```python
from build123d import *

# Parameters (mm, degrees)
F0_R     = 90
F1_DEPTH = 7.5
F2_R     = 3
F3_DEPTH = 90


with BuildPart() as f1:
    # F0 (on Front) → F1 (new body, symmetric)
    with BuildSketch(Plane.XZ):
        Circle(F0_R)
    extrude(amount=F1_DEPTH, both=True)

    # F2 (on Right) → F3 (cut, symmetric)
    with BuildSketch(Plane.YZ):
        Circle(F2_R)
    extrude(amount=F3_DEPTH, both=True, mode=Mode.SUBTRACT)

    # F5 (on Right) → F6 (revolve, cut)
    with BuildSketch(Plane.YZ):
        with BuildLine():
            Line((-7.9027169537, 80), (-7.9027169537, 0))
            Line((-7.9027169537, 0), (-4.3293770832, 0))
            ThreePointArc((-4.3293770832, 0), (-4.580031519, 40.0686088178), (-7.9027169537, 80))
        make_face()
    revolve(axis=Axis((0, 1.0657925159, 0), (0, 1, 0)), mode=Mode.SUBTRACT)


solid = f1.part
```
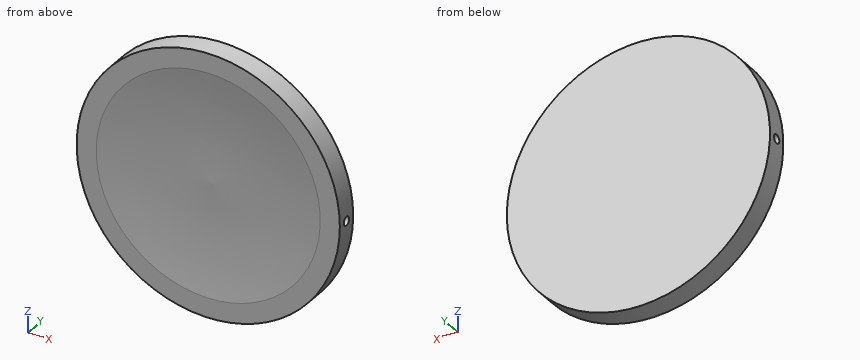
For this review, take the finished solid that the model builds, in its own axes (mm). Coordinates: 2 decimals unless noted, no trailing zeros. Write each loop counter-clockwise with the first axis right and the second up, starting at its lowest first coordinate (ties: lowest second). Pieces come first, ordered by that corner, then holes.
(1) Add section A-A on y = 0. Give the boundary of the cut face in (x, z), then the cut area to 3 significant figures.
(2) Wall thickness on probe 1 along Y at (x, z) = (10, 0); probe 2 along Y at (x, z) = (47.5, 0); probe 3 along Z at (x, y) = (-65, 1.5): over which ranges is each line inside the solid? List them lowest first.
(3) For pin 1 Ø8 at (y, z) = (2, -5.5) entering from +X; pin 2 Ø2 at (y, z) = (-3.5, 17) entering from +X; pin 3 Ø8 at (x, y) = (20.5, -1) entering from -Z, all flat-tipped, find the tip position at first contact; note any pin that passes through.
Answer sheet:
1. outline: (-89.95, -3) arc R90 ccw to (89.95, -3) - close; (-89.95, 3) - (89.95, 3) arc R90 ccw to start
1. area: 24,400 mm2
2. probe 1: y = -4.1 to -3, 3 to 7.5
2. probe 2: y = -4.97 to -3, 3 to 7.5
2. probe 3: z = -62.25 to -2.6, 2.6 to 62.25
3. pin 1: stops at x = 89.99
3. pin 2: stops at x = 88.57
3. pin 3: stops at z = -88.47
